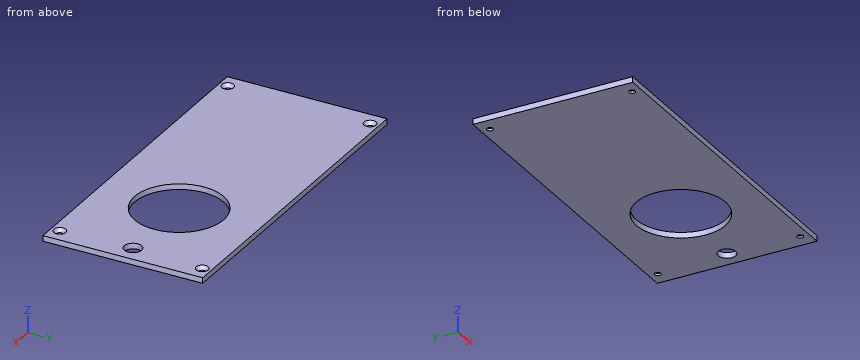
```python
from build123d import *

# Parameters (mm, degrees)
SKETCH1_W                                     = 96
SKETCH1_H                                     = 46
BOSS_EXTRUDE1_DEPTH                           = 1.6002
SKETCH2_R                                     = 12.8397
CUT_EXTRUDE1_DEPTH                            = 2.6002
CSK_FOR_0_FLAT_HEAD_SOCKET_CAP_SCREW1_A_COUNT = 2
CSK_FOR_0_FLAT_HEAD_SOCKET_CAP_SCREW1_A_PITCH = 41
CSK_FOR_0_FLAT_HEAD_SOCKET_CAP_SCRE_2_COUNT   = 2
CSK_FOR_0_FLAT_HEAD_SOCKET_CAP_SCRE_2_PITCH   = 96.629446858
CSK_FOR_0_FLAT_HEAD_SOCKET_CAP_SCRE_3_COUNT   = 2
CSK_FOR_0_FLAT_HEAD_SOCKET_CAP_SCRE_3_PITCH   = 87.5
SKETCH14_R                                    = 2.5
CUT_EXTRUDE2_DEPTH                            = 10


with BuildPart() as part:
    # Sketch1 → Boss-Extrude1 (new body)
    with BuildSketch(Plane.XY):
        with Locations((48, 23)):
            Rectangle(SKETCH1_W, SKETCH1_H)
    extrude(amount=BOSS_EXTRUDE1_DEPTH)

    # Sketch2 → Cut-Extrude1 (cut, through all)
    with BuildSketch(Plane.XY.offset(1.6002)):
        with Locations((66.7, 23)):
            Circle(SKETCH2_R)
    extrude(amount=-CUT_EXTRUDE1_DEPTH, mode=Mode.SUBTRACT)

    # Sketch7 → CSK for #0 Flat Head Socket Cap Screw1 (revolve, cut)
    with BuildSketch(Plane(origin=(4.25, 43.5, 1.6002), x_dir=(0, -1, 0), z_dir=(1, 0, 0))):
        Polygon((0, 0), (0, 1.6002), (0.889, 1.6002), (0.889, 0.993458156), (1.7526, 0), align=None)
    csk_for_0_flat_head_socket_cap_screw1 = revolve(axis=Axis((4.25, 43.5, 7.9502), (0, 0, -1)), mode=Mode.SUBTRACT)

    # CSK for #0 Flat Head Socket Cap Screw1 a: CSK for #0 Flat Head Socket Cap Screw1 ×2
    with Locations(*[(0, -i * CSK_FOR_0_FLAT_HEAD_SOCKET_CAP_SCREW1_A_PITCH, 0) for i in range(1, CSK_FOR_0_FLAT_HEAD_SOCKET_CAP_SCREW1_A_COUNT)]):
        add(csk_for_0_flat_head_socket_cap_screw1, mode=Mode.SUBTRACT)

    # CSK for _0 Flat Head Socket Cap Scre 2: CSK for #0 Flat Head Socket Cap Screw1 ×2
    with Locations(*[Vector(0.905521069, -0.424301301, 0) * (i * CSK_FOR_0_FLAT_HEAD_SOCKET_CAP_SCRE_2_PITCH) for i in range(1, CSK_FOR_0_FLAT_HEAD_SOCKET_CAP_SCRE_2_COUNT)]):
        add(csk_for_0_flat_head_socket_cap_screw1, mode=Mode.SUBTRACT)

    # CSK for _0 Flat Head Socket Cap Scre 3: CSK for #0 Flat Head Socket Cap Screw1 ×2
    with Locations(*[(i * CSK_FOR_0_FLAT_HEAD_SOCKET_CAP_SCRE_3_PITCH, 0, 0) for i in range(1, CSK_FOR_0_FLAT_HEAD_SOCKET_CAP_SCRE_3_COUNT)]):
        add(csk_for_0_flat_head_socket_cap_screw1, mode=Mode.SUBTRACT)

    # Sketch14 → Cut-Extrude2 (cut)
    with BuildSketch(Plane.XY.offset(1.6002)):
        with Locations((90.727040544, 23)):
            Circle(SKETCH14_R)
    extrude(amount=-CUT_EXTRUDE2_DEPTH, mode=Mode.SUBTRACT)


solid = part.part
```
Can you work these out from the model? Positions are in its coordinate system, mm. Coordinates: 2 decimals unless noted, no trailing zeros. Loops run counter-clockwise (first coordinate to the right, second up) from the corner with the lowest first, then second, coordinate; pieces in that order, holes last.
1) Imagine slicing it at A-A on y = 2.5. List the corners of the cut face in (x, z) for me, plus the area to 3 significant figures.
2) Imagine slicing it at C-C on x = 91.75. List the corners of the cut face in (y, z) for me, plus the area to 3 significant figures.
3) Imagine slicing it at D-D on y = 12.5. List the corners of the cut face in (x, z) for me, plus the area to 3 significant figures.
4) For pin 1 (2.5 mm diameter, centred on x = 91.75, y = 2.5, fed in from +Z); pin 2 (1.4 mm diameter, centred on x = 91.75, y = 43.5, fed in from -Z); pin 3 (2 mm diameter, centred on x = 4.25, y = 2.5, fed in from +Z), each with a flat end and sliding along its axis, tell me the tip position at first contact or that it passes through.
5) I need wall thicknesses on probe 1 along Y at (x, z) = (4.25, 0.4); probe 2 along X at (y, z) = (2.5, 0.25); probe 3 along Y at (x, z) = (66.7, 1.1). Which ranges of each line are inside material? Lowest first, please.
6) Imagine slicing it at B-B on x = 4.25. List the corners of the cut face in (y, z) for me.
Completed:
1. outline: (0, 0) - (3.36, 0) - (3.36, 0.61) - (2.5, 1.6) - (0, 1.6) - close; (5.14, 0) - (90.86, 0) - (90.86, 0.61) - (90, 1.6) - (6, 1.6) - (5.14, 0.61) - close; (92.64, 0) - (96, 0) - (96, 1.6) - (93.5, 1.6) - (92.64, 0.61) - close
1. area: 146 mm2
2. outline: (0, 0) - (1.61, 0) - (1.61, 0.61) - (0.75, 1.6) - (0, 1.6) - close; (3.39, 0) - (20.72, 0) - (20.72, 1.6) - (4.25, 1.6) - (3.39, 0.61) - close; (25.28, 0) - (42.61, 0) - (42.61, 0.61) - (41.75, 1.6) - (25.28, 1.6) - close; (44.39, 0) - (46, 0) - (46, 1.6) - (45.25, 1.6) - (44.39, 0.61) - close
2. area: 58.9 mm2
3. outline: (0, 0) - (59.31, 0) - (59.31, 1.6) - (0, 1.6) - close; (74.09, 0) - (96, 0) - (96, 1.6) - (74.09, 1.6) - close
3. area: 130 mm2
4. pin 1: stops at z = 1.02
4. pin 2: passes through
4. pin 3: stops at z = 0.73
5. probe 1: y = 0 to 1.61, 3.39 to 42.61, 44.39 to 46
5. probe 2: x = 0 to 3.36, 5.14 to 90.86, 92.64 to 96
5. probe 3: y = 0 to 10.16, 35.84 to 46
6. outline: (0, 0) - (1.61, 0) - (1.61, 0.61) - (0.75, 1.6) - (0, 1.6) - close; (3.39, 0) - (42.61, 0) - (42.61, 0.61) - (41.75, 1.6) - (4.25, 1.6) - (3.39, 0.61) - close; (44.39, 0) - (46, 0) - (46, 1.6) - (45.25, 1.6) - (44.39, 0.61) - close
